Design review of the part built by this model. Coordinates are the model's own, in mm. A direction names the side the tool comes from. Give positions to 0.01 mm unless a question says otherwise; leave off trailing zeros. Order: outer loops, then holes, each group sorted by start corner. A loop starts at its lowest first (then second) coordinate and runs counter-clockwise, first axis right, second up. Notation, with made-up numbers: (4.25, 41.25) -> (38.25, 41.25) arc R19 ccw to (38.25, 66.25) -> close; hole circle Ø3 at (79.25, -35.5). An arc over 180 degrees is marked (long way). Answer in a Markdown table with one row per item. Add a question column.
```python
from build123d import *

# Parameters (mm, degrees)
BOSS_EXTRUDE1_DEPTH       = 10
FILLET1_R                 = 0.1
FILLET2_R                 = 0.5
SKETCH2_R                 = 1.6
CUT_EXTRUDE1_DEPTH        = 37.455365189
REVISION_INDICATION_DEPTH = 0.4


with BuildPart() as part:
    # Sketch1 → Boss-Extrude1 (new body)
    with BuildSketch(Plane(origin=(0, 0, 0), x_dir=(1, 0, 0), z_dir=(0, 1, 0))):
        Polygon((20.35, 0.7), (14.35, 0.7), (0, 0), (-0.117073171, 2.4), (14.35, 4.3), (20.35, 4.3), (34.817073171, 2.4), (34.7, 0), align=None)
        Polygon((20.35, 2.2), (14.35, 2.2), (0.35, 1.2), (14.35, 2.8), (20.35, 2.8), (34.35, 1.2), align=None, mode=Mode.SUBTRACT)
    extrude(amount=BOSS_EXTRUDE1_DEPTH)

    # Fillet1
    fillet1_edges = [part.edges().sort_by_distance(p)[0] for p in [
        (0.35, 5, -1.2),
        (34.35, 5, -1.2),
    ]]
    fillet(fillet1_edges, radius=FILLET1_R)

    # Fillet2
    fillet2_edges = [part.edges().sort_by_distance(p)[0] for p in [
        (-0.117073171, 5, -2.4),
        (34.817073171, 5, -2.4),
        (34.7, 5, 0),
        (0, 5, 0),
    ]]
    fillet(fillet2_edges, radius=FILLET2_R)

    # Sketch2 → Cut-Extrude1 (cut, through all)
    with BuildSketch(Plane(origin=(0, 0, -4.3), x_dir=(-1, 0, 0), z_dir=(0, 0, -1))):
        with Locations((-17.35, 5)):
            Circle(SKETCH2_R)
    extrude(amount=-CUT_EXTRUDE1_DEPTH, mode=Mode.SUBTRACT)

    # Sketch5 → revision indication (add)
    with BuildSketch(Plane(origin=(-0.311839138, 0, -2.374420857), x_dir=(-0.9914858429395939, 0, 0.13021452780071538), z_dir=(-0.13021452780071538, 0, -0.9914858429395939))):
        with BuildLine():
            add(Edge.make_bspline(
                [(-1.75614285, 1.976923077), (-1.720782037, 1.974821832), (-1.651461296, 1.970702586), (-1.551241734, 1.942442049), (-1.460537137, 1.892261337), (-1.379742922, 1.825381725), (-1.313146886, 1.744291021), (-1.261177847, 1.654309873), (-1.233163488, 1.553251269), (-1.229074248, 1.483528859), (-1.226976184, 1.44775641)],
                knots=[0, 0, 0, 0, 1.020151414, 1.999887582, 2.974338812, 3.990962822, 5.007586832, 5.987933904, 6.967670073, 8, 8, 8, 8], degree=3))
            add(Edge.make_bspline(
                [(-1.226976184, 1.44775641), (-1.229145345, 1.412843512), (-1.233422899, 1.343995789), (-1.261113631, 1.243699421), (-1.313542951, 1.153662038), (-1.379283581, 1.071471016), (-1.46055711, 1.004449722), (-1.551456175, 0.954695939), (-1.651226029, 0.924411918), (-1.720742787, 0.920554208), (-1.75614285, 0.918589744)],
                knots=[0, 0, 0, 0, 1.009421747, 1.99056486, 2.972319754, 3.999869655, 5.017953583, 5.993804169, 6.978383603, 8, 8, 8, 8], degree=3))
            add(Edge.make_bspline(
                [(-1.75614285, 0.918589744), (-1.791568422, 0.920483127), (-1.860728417, 0.924179507), (-1.960125864, 0.955317742), (-2.051578507, 1.003983162), (-2.132836213, 1.071595984), (-2.19912744, 1.153239101), (-2.249247777, 1.244319503), (-2.279347047, 1.343708683), (-2.283305588, 1.412786963), (-2.285309517, 1.44775641)],
                knots=[0, 0, 0, 0, 1.022052826, 1.995314843, 2.982371812, 4.00089066, 5.028879526, 6.005146991, 6.990147033, 8, 8, 8, 8], degree=3))
            add(Edge.make_bspline(
                [(-2.285309517, 1.44775641), (-2.283382565, 1.483587428), (-2.279620429, 1.553543092), (-2.249184588, 1.653690044), (-2.199516318, 1.744709926), (-2.132377959, 1.825258007), (-2.051598165, 1.892726399), (-1.960346478, 1.941829667), (-1.860489026, 1.970931558), (-1.791528138, 1.974891267), (-1.75614285, 1.976923077)],
                knots=[0, 0, 0, 0, 1.032775665, 2.016367738, 2.991239715, 4.008302682, 5.025365648, 6.011011707, 6.979408107, 8, 8, 8, 8], degree=3))
        make_face()
        with BuildLine():
            add(Edge.make_bspline(
                [(-4.117040286, 1.976923077), (-4.081679473, 1.974821832), (-4.012358732, 1.970702586), (-3.91213917, 1.942442049), (-3.821434573, 1.892261337), (-3.740640358, 1.825381725), (-3.674044322, 1.744291021), (-3.622075283, 1.654309873), (-3.594060924, 1.553251269), (-3.589971684, 1.483528859), (-3.587873619, 1.44775641)],
                knots=[0, 0, 0, 0, 1.020151414, 1.999887582, 2.974338812, 3.990962822, 5.007586832, 5.987933904, 6.967670073, 8, 8, 8, 8], degree=3))
            add(Edge.make_bspline(
                [(-3.587873619, 1.44775641), (-3.590042781, 1.412843512), (-3.594320335, 1.343995789), (-3.622011067, 1.243699421), (-3.674440387, 1.153662038), (-3.740181017, 1.071471016), (-3.821454546, 1.004449722), (-3.91235361, 0.954695939), (-4.012123464, 0.924411918), (-4.081640223, 0.920554208), (-4.117040286, 0.918589744)],
                knots=[0, 0, 0, 0, 1.009421747, 1.99056486, 2.972319754, 3.999869655, 5.017953583, 5.993804169, 6.978383603, 8, 8, 8, 8], degree=3))
            add(Edge.make_bspline(
                [(-4.117040286, 0.918589744), (-4.152465858, 0.920483127), (-4.221625853, 0.924179507), (-4.3210233, 0.955317742), (-4.412475943, 1.003983162), (-4.493733649, 1.071595984), (-4.560024876, 1.153239101), (-4.610145213, 1.244319503), (-4.640244483, 1.343708683), (-4.644203024, 1.412786963), (-4.646206953, 1.44775641)],
                knots=[0, 0, 0, 0, 1.022052826, 1.995314843, 2.982371812, 4.00089066, 5.028879526, 6.005146991, 6.990147033, 8, 8, 8, 8], degree=3))
            add(Edge.make_bspline(
                [(-4.646206953, 1.44775641), (-4.644280001, 1.483587428), (-4.640517865, 1.553543092), (-4.610082024, 1.653690044), (-4.560413754, 1.744709926), (-4.493275395, 1.825258007), (-4.412495601, 1.892726399), (-4.321243914, 1.941829667), (-4.221386462, 1.970931558), (-4.152425574, 1.974891267), (-4.117040286, 1.976923077)],
                knots=[0, 0, 0, 0, 1.032775665, 2.016367738, 2.991239715, 4.008302682, 5.025365648, 6.011011707, 6.979408107, 8, 8, 8, 8], degree=3))
        make_face()
        with BuildLine():
            add(Edge.make_bspline(
                [(-6.477937722, 1.976923077), (-6.442576908, 1.974821832), (-6.373256168, 1.970702586), (-6.273036606, 1.942442049), (-6.182332009, 1.892261337), (-6.101537794, 1.825381725), (-6.034941758, 1.744291021), (-5.982972719, 1.654309873), (-5.95495836, 1.553251269), (-5.95086912, 1.483528859), (-5.948771055, 1.44775641)],
                knots=[0, 0, 0, 0, 1.020151414, 1.999887582, 2.974338812, 3.990962822, 5.007586832, 5.987933904, 6.967670073, 8, 8, 8, 8], degree=3))
            add(Edge.make_bspline(
                [(-5.948771055, 1.44775641), (-5.950940217, 1.412843512), (-5.955217771, 1.343995789), (-5.982908503, 1.243699421), (-6.035337823, 1.153662038), (-6.101078453, 1.071471016), (-6.182351982, 1.004449722), (-6.273251046, 0.954695939), (-6.3730209, 0.924411918), (-6.442537658, 0.920554208), (-6.477937722, 0.918589744)],
                knots=[0, 0, 0, 0, 1.009421747, 1.99056486, 2.972319754, 3.999869655, 5.017953583, 5.993804169, 6.978383603, 8, 8, 8, 8], degree=3))
            add(Edge.make_bspline(
                [(-6.477937722, 0.918589744), (-6.513363294, 0.920483127), (-6.582523289, 0.924179507), (-6.681920736, 0.955317742), (-6.773373379, 1.003983162), (-6.854631085, 1.071595984), (-6.920922312, 1.153239101), (-6.971042649, 1.244319503), (-7.001141919, 1.343708683), (-7.00510046, 1.412786963), (-7.007104389, 1.44775641)],
                knots=[0, 0, 0, 0, 1.022052826, 1.995314843, 2.982371812, 4.00089066, 5.028879526, 6.005146991, 6.990147033, 8, 8, 8, 8], degree=3))
            add(Edge.make_bspline(
                [(-7.007104389, 1.44775641), (-7.005177437, 1.483587428), (-7.001415301, 1.553543092), (-6.97097946, 1.653690044), (-6.92131119, 1.744709926), (-6.85417283, 1.825258007), (-6.773393036, 1.892726399), (-6.68214135, 1.941829667), (-6.582283898, 1.970931558), (-6.51332301, 1.974891267), (-6.477937722, 1.976923077)],
                knots=[0, 0, 0, 0, 1.032775665, 2.016367738, 2.991239715, 4.008302682, 5.025365648, 6.011011707, 6.979408107, 8, 8, 8, 8], degree=3))
        make_face()
    extrude(amount=REVISION_INDICATION_DEPTH)


solid = part.part
```
1) Add section A-A, the plane y = 7. Write out the cut boundary in (x, z), and give its area (3 significant figures).
2) Add section B-B, the plane x = 17.35. Write out the cut boundary in (y, z).
3) Add section D-D, the plane x = 7. Write out the cut boundary in (y, z) (3 decimals), and give its area (3 significant figures).
4) Machinability: for faces 4 (the face through (9.763, 4.93, -1.872)), 5 (the face through (15.87, 4.39, -3.56)), 6 (the face through (7.522, 4.93, -0.367)), which of the approach directions +Z, -Z, +X, -X, +Y, -Y give a long, thin tool a straight path to every point of the face, cutting with its end or side? Answer none if there is none.
5) For L1, parallel to Y at x = 17.35, z = -3.75; L2, parallel to Z at x = 19, y = 9.5; L3, parallel to Z at x = 11, y = 1.75, list the stretches that pass through material, from the lowest coordinate up.
6) Mouldability with a two-part tool opening along Z and no side actions: class faces 1 (the face through (9.62, 4.93, -2.26)), 2 (the face through (1.37, 1.46, -3)), 3 (the face through (34.76, 4.93, -1.23)) as +Z half, -Z half, draft (parallel to the pull), parting line (faces both ways), or undercut.
7) Clearance check with flat-ended pins moving along their axes: P1, Ø1.5, axis at x = 11.5, y = 9, coming from the -Z side; P2, Ø1.5, axis at x = 9.5, y = 7, coming from the -Z side; P3, Ø1.8, axis at x = 17, y = 5, coming from the +Z side; P4, Ø3, axis at x = 17, y = 6.5, coming from the +Z side. State where each tip first meets the part, or that it passes through.
8) Add section C-C, the plane y = 5. Write out the cut boundary in (x, z), and give its area (3 significant figures).
Verdict:
| question | item | result |
|---|---|---|
| 1 | outline | (-0.09, -1.94) arc R0.5 ccw to (0.34, -2.46) -> (14.35, -4.3) -> (20.35, -4.3) -> (34.36, -2.46) arc R0.5 ccw to (34.79, -1.94) -> (34.72, -0.5) arc R0.5 ccw to (34.2, -0.02) -> (20.35, -0.7) -> (14.35, -0.7) -> (0.5, -0.02) arc R0.5 ccw to (-0.02, -0.5) -> close; hole (5.03, -1.73) -> (14.35, -2.8) -> (20.35, -2.8) -> (29.67, -1.73) arc R0.1 ccw to (29.66, -1.54) -> (20.35, -2.2) -> (14.35, -2.2) -> (5.04, -1.54) arc R0.1 ccw to start |
| 1 | area | 96.9 mm2 |
| 2 | outline | (0, -4.3) -> (3.4, -4.3) -> (3.4, -2.8) -> (0, -2.8) -> close; (0, -2.2) -> (3.4, -2.2) -> (3.4, -0.7) -> (0, -0.7) -> close; (6.6, -4.3) -> (10, -4.3) -> (10, -2.8) -> (6.6, -2.8) -> close; (6.6, -2.2) -> (10, -2.2) -> (10, -0.7) -> (6.6, -0.7) -> close |
| 3 | outline | (0, -3.335) -> (10, -3.335) -> (10, -1.96) -> (0, -1.96) -> close; (0, -1.675) -> (10, -1.675) -> (10, -0.341) -> (0, -0.341) -> close |
| 3 | area | 27.1 mm2 |
| 4 | face 4 | +Y, -Y |
| 4 | face 5 | +Z, -Z |
| 4 | face 6 | +Z, +Y, -Y |
| 5 | L1 | y = 0 to 3.4, 6.6 to 10 |
| 5 | L2 | z = -4.3 to -2.8, -2.2 to -0.7 |
| 5 | L3 | z = -3.86 to -2.42, -1.96 to -0.54 |
| 6 | face 1 | undercut |
| 6 | face 2 | -Z half |
| 6 | face 3 | +Z half |
| 7 | P1 | stops at z = -4.02 |
| 7 | P2 | stops at z = -3.76 |
| 7 | P3 | passes through |
| 7 | P4 | stops at z = -0.7 |
| 8 | outline | (-0.09, -1.94) arc R0.5 ccw to (0.34, -2.46) -> (14.35, -4.3) -> (15.75, -4.3) -> (15.75, -2.8) -> (14.35, -2.8) -> (5.03, -1.73) arc R0.1 cw to (5.04, -1.54) -> (14.35, -2.2) -> (15.75, -2.2) -> (15.75, -0.7) -> (14.35, -0.7) -> (0.5, -0.02) arc R0.5 ccw to (-0.02, -0.5) -> close; (18.95, -4.3) -> (20.35, -4.3) -> (34.36, -2.46) arc R0.5 ccw to (34.79, -1.94) -> (34.72, -0.5) arc R0.5 ccw to (34.2, -0.02) -> (20.35, -0.7) -> (18.95, -0.7) -> (18.95, -2.2) -> (20.35, -2.2) -> (29.66, -1.54) arc R0.1 cw to (29.67, -1.73) -> (20.35, -2.8) -> (18.95, -2.8) -> close |
| 8 | area | 87.3 mm2 |
